```python
from build123d import *

# Parameters (mm, degrees)
SKETCH_1_W          = 20
SKETCH_1_H          = 20
SKETCH_1_W_2        = 17
SKETCH_1_H_2        = 17
EXTRUDE_1_DEPTH     = 110
SKETCH_2_R          = 2.7
CUT_EXTRUDE_1_DEPTH = 25
SKETCH_3_R          = 2
CUT_EXTRUDE_2_DEPTH = 20
SKETCH_5_R          = 5
CUT_EXTRUDE_4_DEPTH = 10
CUT_EXTRUDE_START   = -10
SKETCH_6_R          = 5
CUT_EXTRUDE_5_DEPTH = 10


with BuildPart() as part:
    # ｽｹｯﾁ1 → ﾎﾞｽ - 押し出し1 (new body)
    with BuildSketch(Plane.XY):
        Rectangle(SKETCH_1_W, SKETCH_1_H)
        Rectangle(SKETCH_1_W_2, SKETCH_1_H_2, mode=Mode.SUBTRACT)
    extrude(amount=EXTRUDE_1_DEPTH)

    # ｽｹｯﾁ2 → ｶｯﾄ - 押し出し1 (cut)
    with BuildSketch(Plane(origin=(10, 0, 0), x_dir=(0, 0, -1), z_dir=(1, 0, 0))):
        with Locations((-60, 0)):
            Circle(SKETCH_2_R)
        with Locations((-10, 0)):
            Circle(SKETCH_2_R)
    extrude(amount=-CUT_EXTRUDE_1_DEPTH, mode=Mode.SUBTRACT)

    # ｽｹｯﾁ3 → ｶｯﾄ - 押し出し2 (cut)
    with BuildSketch(Plane(origin=(0, 10, 0), x_dir=(1, 0, 0), z_dir=(0, 1, 0))):
        with Locations((0, -100)):
            Circle(SKETCH_3_R)
        with Locations((0, -80)):
            Circle(SKETCH_3_R)
        with Locations((0, -20)):
            Circle(SKETCH_3_R)
    extrude(amount=-CUT_EXTRUDE_2_DEPTH, mode=Mode.SUBTRACT)

    # ｽｹｯﾁ5 → ｶｯﾄ - 押し出し4 (cut)
    with BuildSketch(Plane(origin=(0, -10, 0), x_dir=(-1, 0, 0), z_dir=(0, -1, 0))):
        with Locations((0, -20)):
            Circle(SKETCH_5_R)
    extrude(amount=-CUT_EXTRUDE_4_DEPTH, mode=Mode.SUBTRACT)

    # ｽｹｯﾁ6 → ｶｯﾄ - 押し出し5 (cut)
    with BuildSketch(Plane.ZY.offset(10).offset(CUT_EXTRUDE_START)):
        with Locations((10, 0)):
            Circle(SKETCH_6_R)
        with Locations((60, 0)):
            Circle(SKETCH_6_R)
    extrude(amount=-CUT_EXTRUDE_5_DEPTH, mode=Mode.SUBTRACT)


solid = part.part
```
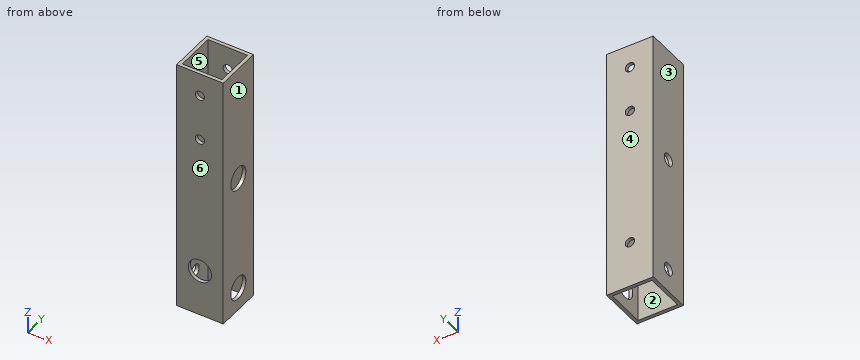
Could you check a few things on this model? Use its own coordinates, in mm. Face numbers are marked on the shaded views. A direction names the side the tool comes from. Coordinates: 2 decimals unless noted, no trailing zeros. Order: outer loops, then holes, each group sorted by start corner. A loop starts at its lowest first (then second) coordinate and runs counter-clockwise, first axis right, second up. Notation, with made-up numbers: M 66,-17 L 102,-17 A15 ccw 102,-6 Z; hole C -12.5,51 d3. An arc over 180 degrees is marked long. Use a Markdown table: item, result. Add a question column.
Q1. I want a section at A-A on z = 10. List the corners of the cut face in (x, y) for me.
Q2. We'd pull the mould along Y, two halves only. Please class the marked faces 3, 4, 5 and 6: pulls with the +Y half, pulls with the -Y half, needs draft (parallel to the pull), parting line crosses it, or undercut.
Q3. I want a section at D-D on x = 0. Give the number of separate pieces and of enclosed holes in the cut face, then the cut area to 3 significant figures.
Q4. Which directions (+Z, -Z, +X, -X, +Y, -Y) give clear straight access to the entire face, cutting with the end or side of a thin tool? Please do the marked faces 1 and 2.
Q5. I want a section at B-B on x = 6.25. List the corners of the cut face in (y, z) for me, then the cut area to 3 significant figures.
Q6. I'm going to push flat-ended pins straight in: pin 1 (3.5 mm diameter, centred on x = 0, z = 100, fed in from -Y); pin 2 (9 mm diameter, centred on x = 0, z = 20, fed in from -Y). Where does each tip first touch, or does it pass through?
Q7. If I drill on L1, parallel to Z at x = 0, y = -9.55; L2, parallel to Z at x = 0, y = 9; L3, parallel to Y at x = 7, z = 8, over which ranges is the centre line in solid material (lowest first)?
Checked values:
| question | item | result |
|---|---|---|
| 1 | outline | M -10,-10 L 10,-10 L 10,-5 L 8.5,-5 L 8.5,-8.5 L -8.5,-8.5 L -8.5,-2.7 L -10,-2.7 Z; M -10,2.7 L -8.5,2.7 L -8.5,8.5 L 8.5,8.5 L 8.5,5 L 10,5 L 10,10 L -10,10 Z |
| 2 | face 3 | needs draft |
| 2 | face 4 | pulls with the +Y half |
| 2 | face 5 | undercut |
| 2 | face 6 | pulls with the -Y half |
| 3 | separate pieces | 8 |
| 3 | enclosed holes | 0 |
| 3 | area | 285 mm² |
| 4 | face 1 | +Z, -Z, +X, +Y, -Y |
| 4 | face 2 | +Z, -Z |
| 5 | outline | M -10,0 L -8.5,0 L -8.5,110 L -10,110 Z; M 8.5,0 L 10,0 L 10,110 L 8.5,110 Z |
| 5 | area | 330 mm² |
| 6 | pin 1 | through |
| 6 | pin 2 | y = 8.5 |
| 7 | L1 | 0 to 15, 25 to 78, 82 to 98, 102 to 110 |
| 7 | L2 | 0 to 18, 22 to 78, 82 to 98, 102 to 110 |
| 7 | L3 | -10 to -8.5, 8.5 to 10 |
